Verification items for the finished model (mm, model axes). Coordinates: 2 decimals unless noted, no trailing zeros. Order: outer loops, then holes, each group sorted by start corner. A loop starts at its lowest first (then second) coordinate and runs counter-clockwise, first axis right, second up. Notation, with made-up numbers: M 43,21 L 90,21 A20 ccw 90,30 Z; hole C 44.25,29.25 d11. An arc over 180 degrees is marked long. Return JSON: item names as keys, results as strings. Group by question number.
Q1. Section check C-C, the plane z = 0.4. Enter the section's corners in (x, y), then the cut area to 3 significant figures.
Q2. Section check B-B, the plane x = 0. Enter the section's corners in (y, z), then the cut area to 3 significant figures.
Q3. Mould release check, pull along X, two halves, no side actions. Record for faces 1 (the face through (6.466, -2.681, 0.493)), 2 (the face through (0, 0, 1)): pulls with the +X half, pulls with the -X half, needs draft (parallel to the pull), parting line crosses it, or undercut.
Q4. Section check D-D, the plane x = -5.5. Enter the section's corners in (y, z).
Q5. Section check A-A, the plane y = 0. Enter the section's corners in (x, z).
Q6. Thickness scan on probe 1 along X at (y, z) = (-1, -0.2); probe 2 along Y at (x, z) = (-2, -0.25); probe 3 along Z at (x, y) = (0, 5.25). Record the ranges inside material, lowest first.
Q7. Go/stop test with flat-tipped pins: pin 1 Ø1.5 at (x, y) = (-1.5, -7.5) entering from +Z; pin 2 Ø3 at (x, y) = (-3, -8.5) entering from +Z. Record where each tip stops, or that it passes through.
from build123d import *

# Parameters (mm, degrees)
SKETCH1_R           = 7
BOSS_EXTRUDE1_DEPTH = 1
SKETCH2_W           = 10
SKETCH2_H           = 14
BOSS_EXTRUDE2_DEPTH = 0.5


with BuildPart() as part:
    # Sketch1 → Boss-Extrude1 (new body)
    with BuildSketch(Plane.XY):
        Circle(SKETCH1_R)
    extrude(amount=BOSS_EXTRUDE1_DEPTH)

    # Sketch2 → Boss-Extrude2 (add)
    with BuildSketch(Plane(origin=(0, 0, 0), x_dir=(-1, 0, 0), z_dir=(0, 0, -1))):
        with Locations((0, -3)):
            Rectangle(SKETCH2_W, SKETCH2_H)
    extrude(amount=BOSS_EXTRUDE2_DEPTH)


solid = part.part
Numbers:
{
 "1": {"outline": "C 0,0 d14", "area": "154 mm2"},
 "2": {"outline": "M -10,-0.5 L 4,-0.5 L 4,0 L 7,0 L 7,1 L -7,1 L -7,0 L -10,0 Z", "area": "21.0 mm2"},
 "3": {"face 1": "parting line crosses it", "face 2": "needs draft"},
 "4": {"outline": "M -4.33,0 L 4.33,0 L 4.33,1 L -4.33,1 Z"},
 "5": {"outline": "M -7,0 L -5,0 L -5,-0.5 L 5,-0.5 L 5,0 L 7,0 L 7,1 L -7,1 Z"},
 "6": {"probe 1": "x = -5 to 5", "probe 2": "y = -10 to 4", "probe 3": "z = 0 to 1"},
 "7": {"pin 1": "stops at z = 1", "pin 2": "stops at z = 0"}
}
